from build123d import *

# Parameters (mm, degrees)
ESQUISSE1_R        = 1.25
ESQUISSE1_R_2      = 2.25
ESQUISSE1_R_3      = 1.75
ESQUISSE1_W        = 20
ESQUISSE1_H        = 20
ESQUISSE1_W_2      = 6
ESQUISSE1_H_2      = 3
ESQUISSE1_W_3      = 3
ESQUISSE1_H_3      = 6
BOSS_EXTRU_1_DEPTH = 5


with BuildPart() as part:
    # Esquisse1 → Boss.-Extru.1 (new body)
    with BuildSketch(Plane.XY):
        with BuildLine():
            Line((0, 0), (150, 0))
            Line((150, 0), (150, -100))
            ThreePointArc((150, -100), (144.142135624, -114.142135624), (130, -120))
            Line((130, -120), (20, -120))
            ThreePointArc((20, -120), (5.857864376, -114.142135624), (0, -100))
            Line((0, -100), (0, 0))
        make_face()
        with Locations((90, -44)):
            Circle(ESQUISSE1_R, mode=Mode.SUBTRACT)
        with Locations((139, -44)):
            Circle(ESQUISSE1_R, mode=Mode.SUBTRACT)
        with Locations((139, -102)):
            Circle(ESQUISSE1_R, mode=Mode.SUBTRACT)
        with Locations((90, -102)):
            Circle(ESQUISSE1_R, mode=Mode.SUBTRACT)
        with Locations((8.5, -31)):
            Circle(ESQUISSE1_R_2, mode=Mode.SUBTRACT)
        with Locations((141.5, -31)):
            Circle(ESQUISSE1_R_2, mode=Mode.SUBTRACT)
        with Locations((25, -10)):
            Circle(ESQUISSE1_R_2, mode=Mode.SUBTRACT)
        with Locations((125, -10)):
            Circle(ESQUISSE1_R_2, mode=Mode.SUBTRACT)
        with Locations((96, -30)):
            Circle(ESQUISSE1_R_2, mode=Mode.SUBTRACT)
        with Locations((54, -30)):
            Circle(ESQUISSE1_R_2, mode=Mode.SUBTRACT)
        with Locations((75, -10)):
            Circle(ESQUISSE1_R_2, mode=Mode.SUBTRACT)
        with Locations((11.5, -97.5)):
            Circle(ESQUISSE1_R_3, mode=Mode.SUBTRACT)
        with Locations((59.76, -97.5)):
            Circle(ESQUISSE1_R_3, mode=Mode.SUBTRACT)
        with Locations((44.52, -47)):
            Circle(ESQUISSE1_R_3, mode=Mode.SUBTRACT)
        with Locations((75, -30)):
            Rectangle(ESQUISSE1_W, ESQUISSE1_H, mode=Mode.SUBTRACT)
        with Locations((8.5, -35.5)):
            Rectangle(ESQUISSE1_W_2, ESQUISSE1_H_2, mode=Mode.SUBTRACT)
        with Locations((8.5, -21.5)):
            Rectangle(ESQUISSE1_W_2, ESQUISSE1_H_2, mode=Mode.SUBTRACT)
        with Locations((141.5, -35.5)):
            Rectangle(ESQUISSE1_W_2, ESQUISSE1_H_2, mode=Mode.SUBTRACT)
        with Locations((141.5, -21.5)):
            Rectangle(ESQUISSE1_W_2, ESQUISSE1_H_2, mode=Mode.SUBTRACT)
        with Locations((100.6, -30)):
            Rectangle(ESQUISSE1_W_3, ESQUISSE1_H_3, mode=Mode.SUBTRACT)
        with Locations((86.6, -30)):
            Rectangle(ESQUISSE1_W_3, ESQUISSE1_H_3, mode=Mode.SUBTRACT)
        with Locations((49.4, -30)):
            Rectangle(ESQUISSE1_W_3, ESQUISSE1_H_3, mode=Mode.SUBTRACT)
        with Locations((63.4, -30)):
            Rectangle(ESQUISSE1_W_3, ESQUISSE1_H_3, mode=Mode.SUBTRACT)
    extrude(amount=BOSS_EXTRU_1_DEPTH)


solid = part.part
Can you work these out from the model? Positions are in its coordinate system, mm. A direction names the side the tool comes from. Round coordinates to 2 decimals unless told otherwise and drop trailing zeros. Order: outer loops, then holes, each group sorted by start corner. A loop starts at its lowest first (then second) coordinate and runs counter-clockwise, first axis right, second up. Notation, with made-up numbers: (-22, 26) -> (6, 26) arc R18 ccw to (6, 49) -> close; hole circle Ø11 at (-0.5, -16.5). An arc over 180 degrees is marked (long way). Write each question's results on one line, items separated by ' | '. Start each with the question number.
Item 1: Will this pin go through, and if not, where does the flat tip stop? pin 1 (3.5 mm diameter, centred on x = 75, y = -10, fed in from -Z).
Item 2: Thinking about a two-plate mould opening in X: for faces 1 (the flat face through (138.5, -22, 2)), 2 (the flat face through (0, -51, 2)), 3 (the flat face through (76, -59, 5)), which applies, +X half, -X half, draft (parallel to the pull), parting line (faces both ways), or undercut?
Item 3: Please list where these lines run through material, in increasing order: L1, parallel to Y at x = 90, z = 3.55; L2, parallel to Y at x = 80, z = 3.1; L3, parallel to Y at x = 139, z = 3.4.
Item 4: If we section it at C-C, the plane x = 44.52: Write out the boundary of the cut face in (y, z), then the cut area to 4 significant figures.
Item 5: If we section it at B-B, the plane y = -97.5: Write out the boundary of the cut face in (x, z), then the cut area to 3 significant figures.
Item 6: Which directions (+Z, -Z, +X, -X, +Y, -Y) give clear straight access to the entire face, cutting with the end or side of a thin tool? Please do faces 4 (the cylindrical face through (6.014, -114.297, 2.465)), 5 (the flat face through (11.5, -36, 2)).
Item 7: If we section it at A-A, the plane x = 80.5: Write out the boundary of the cut face in (y, z), then the cut area to 3 significant figures.
Item 8: If we section it at D-D, the plane z = 3.5: State how many separate pieces and enclosed holes the cut face has, then the cut area to 3 significant figures.
Results:
1) pin 1: passes through
2) face 1: undercut | face 2: -X half | face 3: draft
3) L1: y = -120 to -103.25, -100.75 to -45.25, -42.75 to 0 | L2: y = -120 to -40, -20 to 0 | L3: y = -117.86 to -103.25, -100.75 to -45.25, -42.75 to -37, -34 to -23, -20 to 0
4) outline: (-120, 0) -> (-48.75, 0) -> (-48.75, 5) -> (-120, 5) -> close; (-45.25, 0) -> (0, 0) -> (0, 5) -> (-45.25, 5) -> close | area: 582.5 mm2
5) outline: (0, 0) -> (9.75, 0) -> (9.75, 5) -> (0, 5) -> close; (13.25, 0) -> (58.01, 0) -> (58.01, 5) -> (13.25, 5) -> close; (61.51, 0) -> (150, 0) -> (150, 5) -> (61.51, 5) -> close | area: 715 mm2
6) face 4: +Z, -Z, -X, -Y | face 5: +Z, -Z
7) outline: (-120, 0) -> (-40, 0) -> (-40, 5) -> (-120, 5) -> close; (-20, 0) -> (0, 0) -> (0, 5) -> (-20, 5) -> close | area: 500 mm2
8) separate pieces: 1 | enclosed holes: 23 | area: 17,100 mm2
